Here's how the part is built. I have some questions about the finished solid (model axes, mm). A direction names the side the tool comes from. Round coordinates to 2 decimals unless told otherwise and drop trailing zeros. Order: outer loops, then holes, each group sorted by start corner. A loop starts at its lowest first (then second) coordinate and runs counter-clockwise, first axis right, second up. Notation, with made-up numbers: (71, 73.5) - (109, 73.5) arc R19 ccw to (109, 101.5) - close; hole circle Ø8 at (-29, 44.25). An arc over 180 degrees is marked (long way). One line per item, written item: value.
from build123d import *

# Parameters (mm, degrees)
F0_W      = 80.264
F0_H      = 101.6
F1_DEPTH  = 2.54
F2_R      = 3.81
F3_W      = 72.644
F3_H      = 93.98
F4_DEPTH  = 1.27
F5_W      = 23.8125
F5_H      = 31.75
F6_DEPTH  = 1.27
F7_W      = 23.8125
F7_H      = 31.75
F8_DEPTH  = 1.27
F9_R      = 2.7305
F10_DEPTH = 1.27
F12_D     = 3.175
F12_DEPTH = 9.525
F12_TIP   = 0.9538662327


with BuildPart() as f1:
    # F0 (on Front) → F1 (new body, symmetric)
    with BuildSketch(Plane.XZ):
        Rectangle(F0_W, F0_H)
    extrude(amount=F1_DEPTH, both=True)

    # F2
    f2_edges = [f1.edges().sort_by_distance(p)[0] for p in [
        (-40.132, 0, 50.8),
        (40.132, 0, 50.8),
        (40.132, 0, -50.8),
        (-40.132, 0, -50.8),
    ]]
    fillet(f2_edges, radius=F2_R)

    # F3 (on face) → F4 (cut)
    with BuildSketch(Plane.XZ.offset(2.54)):
        Rectangle(F3_W, F3_H)
    extrude(amount=-F4_DEPTH, mode=Mode.SUBTRACT)

    # F5 (on face) → F6 (cut, symmetric)
    with BuildSketch(Plane.XZ.offset(1.27)):
        with Locations((-17.5078902394, 22.415274836)):
            Rectangle(F5_W, F5_H)
        with Locations((17.5078902394, 22.415274836)):
            Rectangle(F5_W, F5_H)
    extrude(amount=F6_DEPTH, both=True, mode=Mode.SUBTRACT)

    # F7 (on face) → F8 (cut, symmetric)
    with BuildSketch(Plane.XZ.offset(1.27)):
        with Locations((-17.5078902394, -21.8638093457)):
            Rectangle(F7_W, F7_H)
        with Locations((17.5078902394, -21.8638093457)):
            Rectangle(F7_W, F7_H)
    extrude(amount=F8_DEPTH, both=True, mode=Mode.SUBTRACT)

    # F9 (on face) → F10 (cut)
    with BuildSketch(Plane.XZ.offset(1.27)):
        with Locations((-5.6016402394, 38.290274836)):
            Circle(F9_R)
        with Locations((-5.6016402394, -5.9888093457)):
            Circle(F9_R)
        with Locations((5.6016402394, 38.290274836)):
            Circle(F9_R)
        with Locations((5.6016402394, -5.9888093457)):
            Circle(F9_R)
    extrude(amount=-F10_DEPTH, mode=Mode.SUBTRACT)

    # F12
    with Locations(Plane(origin=(0, 2.54, 0), x_dir=(-1, 0, 0), z_dir=(0, 1, 0))):
        with Locations((-36.322, 46.99), (36.322, 46.99), (36.322, -46.99), (-36.322, -46.99)):
            Hole(F12_D / 2, depth=F12_DEPTH)
            with Locations((0, 0, -(F12_DEPTH + F12_TIP / 2))):  # 118° drill point
                Cone(0, F12_D / 2, F12_TIP, mode=Mode.SUBTRACT)


solid = f1.part
Q1. If we section it at C-C, the plane x = 7: Please give me the cut outline in (y, z), then the cut area to 3 significant figures.
Results list:
outline: (-2.54, -50.8) - (2.54, -50.8) - (2.54, 50.8) - (-2.54, 50.8) - (-2.54, 46.99) - (-1.27, 46.99) - (-1.27, 40.64) - (0, 40.64) - (0, 6.54) - (-1.27, 6.54) - (-1.27, -3.64) - (0, -3.64) - (0, -37.74) - (-1.27, -37.74) - (-1.27, -46.99) - (-2.54, -46.99) - close
area: 310 mm²
Q2. If we section it at A-A, the plane z = 5: Please give me the cut outline in (x, y), then the cut area to 3 significant figures.
Results list:
outline: (-40.13, -2.54) - (-36.32, -2.54) - (-36.32, -1.27) - (36.32, -1.27) - (36.32, -2.54) - (40.13, -2.54) - (40.13, 2.54) - (-40.13, 2.54) - close
area: 315 mm²
Q3. If I drill on line 1 along Z through (x, y) = (-15.5, -0.75); line 2 along X through (y, z) = (-1.15, 46.99); line 3 along X through (y, z) = (-0.9, -14.5), over which ranges is the centre line in solid material (lowest first)?
Results list:
line 1: -50.8 to -37.74, -5.99 to 6.54, 38.29 to 50.8
line 2: -40.13 to -37.91, -34.73 to 34.73, 37.91 to 40.13
line 3: -40.13 to -29.41, -5.6 to 5.6, 29.41 to 40.13
Q4. Will these pins go through, and if not, where does the flat tip stop? pin 1 (12 mm diameter, centred on x = 12.5, z = -2, fed in from -Y); pin 2 (4.5 mm diameter, centred on x = -5.6, z = -5.99, fed in from -Y); pin 3 (1.9 mm diameter, centred on x = -36.322, z = -46.99, fed in from -Y).
Results list:
pin 1: y = -1.27
pin 2: y = 0
pin 3: through
Q5. Which directions (+Z, -Z, +X, -X, +Y, -Y) give clear straight access to the entire face, cutting with the end or side of a thin tool? Please do faces 1 (the cylindrical face through (-3.61, -0.64, 40.16)), 2 (the cylindrical face through (-37.492, -0.036, 48.063)).
Results list:
face 1: -Y
face 2: +Y, -Y
Q6. If we section it at B-B, the plane x = -28: Please give me the cut outline in (y, z).
Results list:
outline: (-2.54, -50.8) - (2.54, -50.8) - (2.54, 50.8) - (-2.54, 50.8) - (-2.54, 46.99) - (-1.27, 46.99) - (-1.27, 38.29) - (0, 38.29) - (0, 6.54) - (-1.27, 6.54) - (-1.27, -5.99) - (0, -5.99) - (0, -37.74) - (-1.27, -37.74) - (-1.27, -46.99) - (-2.54, -46.99) - close
Q7. We'd pull the mould along X, two halves only. Please class faces 3 (the cylindrical face through (39, 0, 49.7)), 4 (the flat face through (16, 0, 24)), 5 (the flat face through (-39, -2.54, 0)), 6 (the flat face through (16, 0, -20)): released by +X, released by -X, zero draft, split by the parting line, or undercut.
Results list:
face 3: released by +X
face 4: undercut
face 5: zero draft
face 6: undercut
